Geometry check sheet. Reference: the model listing, model coordinates, mm. A direction names the side the tool comes from. Give positions to 0.01 mm unless a question says otherwise; leave off trailing zeros. Write each loop counter-clockwise with the first axis right and the second up, starting at its lowest first coordinate (ties: lowest second). Pieces come first, ordered by that corner, then holes. Notation, with made-up numbers: (51.5, 20) - (60.5, 20) arc R33 ccw to (60.5, 48) - close; hole circle Ø8 at (-0.5, -1.75). An arc over 180 degrees is marked (long way). Use a Markdown table: item, result.
```python
from build123d import *

# Parameters (mm, degrees)
SKETCH011_W             = 160
SKETCH011_H             = 60
SKETCH011_R             = 1.2
SKETCH011_W_2           = 27.5
SKETCH011_H_2           = 31.5
PAD004_DEPTH            = 4
SKETCH012_W             = 151.8
SKETCH012_H             = 51.8
SKETCH012_W_2           = 147.8
SKETCH012_H_2           = 47.8
PAD005_DEPTH            = 30
SKETCH013_W             = 160
SKETCH013_H             = 60
SKETCH013_W_2           = 151.8
SKETCH013_H_2           = 51.8
PAD006_DEPTH            = 20
SKETCH014_W             = 20.2
SKETCH014_H             = 5
POCKET004_DEPTH         = 27
SKETCH027_R             = 1.2
POCKET014_DEPTH         = 160.001
POCKET015_DEPTH         = 30.001
LINEARPATTERN007_COUNT  = 5
LINEARPATTERN007_PITCH  = 9
BODY002_PLACEMENT_ANGLE = 180


with BuildPart() as part:
    # Sketch011 → Pad004 (new body)
    with BuildSketch(Plane.YZ):
        with Locations((0, 30)):
            Rectangle(SKETCH011_W, SKETCH011_H)
        with Locations((22, 23.75)):
            Circle(SKETCH011_R, mode=Mode.SUBTRACT)
        with Locations((58, 23.75)):
            Circle(SKETCH011_R, mode=Mode.SUBTRACT)
        with Locations((40, 23.75)):
            Rectangle(SKETCH011_W_2, SKETCH011_H_2, mode=Mode.SUBTRACT)
    extrude(amount=PAD004_DEPTH)

    # Sketch012 → Pad005 (join)
    with BuildSketch(Plane.YZ):
        with Locations((0, 30)):
            Rectangle(SKETCH012_W, SKETCH012_H)
        with Locations((0, 30)):
            Rectangle(SKETCH012_W_2, SKETCH012_H_2, mode=Mode.SUBTRACT)
    extrude(amount=PAD005_DEPTH)

    # Sketch013 → Pad006 (join)
    with BuildSketch(Plane.YZ):
        with Locations((0, 30)):
            Rectangle(SKETCH013_W, SKETCH013_H)
        with Locations((0, 30)):
            Rectangle(SKETCH013_W_2, SKETCH013_H_2, mode=Mode.SUBTRACT)
    extrude(amount=PAD006_DEPTH)

    # Sketch014 (on DatumPlane) → Pocket004 (cut)
    with BuildSketch(Plane.XZ.offset(-80)):
        with Locations((14.1, 53.5)):
            Rectangle(SKETCH014_W, SKETCH014_H)
    extrude(amount=POCKET004_DEPTH, mode=Mode.SUBTRACT)

    # Sketch027 (on DatumPlane) → Pocket014 (cut, through all)
    with BuildSketch(Plane.XZ.offset(-80)):
        with Locations((25, 28)):
            Circle(SKETCH027_R)
    extrude(amount=POCKET014_DEPTH, mode=Mode.SUBTRACT)

    # Sketch028 → Pocket015 (cut, through all)
    with BuildSketch(Plane.YZ):
        with BuildLine():
            Line((6, 11.5), (-64, 11.5))
            ThreePointArc((-64, 11.5), (-65.5, 10), (-64, 8.5))
            Line((6, 8.5), (-64, 8.5))
            ThreePointArc((6, 8.5), (7.5, 10), (6, 11.5))
        make_face()
    pocket015 = extrude(amount=POCKET015_DEPTH, mode=Mode.SUBTRACT)

    # LinearPattern007: Pocket015 ×5
    with Locations(*[(0, 0, i * LINEARPATTERN007_PITCH) for i in range(1, LINEARPATTERN007_COUNT)]):
        add(pocket015, mode=Mode.SUBTRACT)


with BuildPart() as part_1:
    # Body002 placement: moved
    add(part.part.moved(Location((200, 0, -4))).rotate(Axis((200, 0, -4), (0, 0, 1)), BODY002_PLACEMENT_ANGLE))


solid = part_1.part
```
1) Section check D-D on z = 30. Record the boundary of the cut face in (x, y), then the cut area to 3 significant figures.
Working result:
| item | result |
|---|---|
| outline | (170, -75.9) - (180, -75.9) - (180, -80) - (200, -80) - (200, -53.75) - (196, -53.75) - (196, -73.9) - (170, -73.9) - close; (170, 73.9) - (196, 73.9) - (196, -26.25) - (200, -26.25) - (200, 80) - (180, 80) - (180, 75.9) - (170, 75.9) - close |
| area | 765 mm² |
2) Section check B-B on z = 15. Record the boundary of the cut face in (x, y), then the cut area to 3 significant figures.
Working result:
| item | result |
|---|---|
| outline | (170, -75.9) - (180, -75.9) - (180, -80) - (200, -80) - (200, -53.75) - (196, -53.75) - (196, -73.9) - (170, -73.9) - close; (170, 73.9) - (196, 73.9) - (196, 65.5) - (200, 65.5) - (200, 80) - (180, 80) - (180, 75.9) - (170, 75.9) - close; (196, -26.25) - (200, -26.25) - (200, -7.5) - (196, -7.5) - close |
| area | 473 mm² |
3) Section check C-C on y = -62.5. Record the boundary of the cut face in (x, z).
Working result:
| item | result |
|---|---|
| outline | (170, 0.1) - (180, 0.1) - (180, -4) - (200, -4) - (200, 56) - (180, 56) - (180, 52) - (196, 52) - (196, 2.1) - (170, 2.1) - close; (170, 49.9) - (175.8, 49.9) - (175.8, 51.9) - (170, 51.9) - close |
4) Section check A-A on y = 9.5. Count the separate pieces of the cut face and the enclosed holes in it, then the cut area to 3 significant figures.
Working result:
| item | result |
|---|---|
| separate pieces | 6 |
| enclosed holes | 0 |
| area | 415 mm² |
5) Set-up check for faces 4 (the flat face through (198, 29, 22.5)), 5 (the flat face through (175.8, -65, 51)), 6 (the flat face through (183, 73.9, 26)): record each of +Z, -Z, +X, -X, +Y, -Y from which the full face is reachable in a straight line by a thin tool's end or side.
Working result:
| item | result |
|---|---|
| face 4 | +X, -X |
| face 5 | +Z, -Y |
| face 6 | -X |
6) Material ranges on L1, parallel to Z at x = 196.8, y = -22; L2, parallel to Y at x = 180.75, z = 21.5; L3, parallel to Y at x = 175.75, z = 35, recorded low to high. Write a range as from..to.
Working result:
| item | result |
|---|---|
| L1 | z = -4..18.55, 20.95..56 |
| L2 | y = -80..-73.9, 73.9..80 |
| L3 | y = -75.9..-73.9, 73.9..75.9 |
7) Mould release check, pull along Y, two halves, no side actions. Record for faces 1 (the flat face through (190, 1, 56)), 2 (the flat face through (190, -80, 26)), 3 (the flat face through (198, 29, 4.5)): pulls with the +Y half, pulls with the -Y half, needs draft (parallel to the pull), parting line crosses it, or undercut.
Working result:
| item | result |
|---|---|
| face 1 | needs draft |
| face 2 | pulls with the -Y half |
| face 3 | undercut |
8) Depth check by flat-ended pin: P1, Ø1, axis at x = 174.5, z = 13, coming from the +Y side; P2, Ø18, axis at y = -1, z = 20, coming from the -X side; P3, Ø4, axis at x = 173.5, y = 34, coming from the +Z side. Enter the tip coordinate at first touch or a pass-through.
Working result:
| item | result |
|---|---|
| P1 | stops at y = 75.9 |
| P2 | stops at x = 196 |
| P3 | stops at z = 51.9 |
